Can you work these out from the drawing? Everything is in mm from the part's minimum corner. Round coordinates to 2 decimals unless told otherwise and drop trailing zeros. Order: outer loops, then holes, each group sorted by start corner. A loop starts at its lowest first (then second) coordinate and runs counter-clockwise, first axis right, second up. Notation, with made-up numbers: M 13.5,9.5 L 25.5,9.5 A15 cw 25.5,30.5 Z; hole C 62.25,70 d3. An arc over 180 degrees is marked long. Write item = value, one per line. Start each with the question number.
Item 1: I want a section at B-B, the plane x = 216. List the corners of the cut face in (y, z) for me.
Item 2: I want a section at C-C, the plane y = 1.8. List the corners of the cut face in (x, z) for me (3 decimals).
Item 3: I want a section at A-A, the plane z = 80. List the corners of the cut face in (x, y) for me (3 decimals), plus the area to 3 significant figures.
Item 4: I'm going to push flat-ended pins straight in: P1, Ø1.5, axis at x = 214.5, y = 2.5, coming from the +Z side; P2, Ø0.9, axis at x = 92.5, y = 2, coming from the +Z side. Where does each tip first touch, or does it pass through?
Item 5: I want a section at D-D, the plane x = 57.5. List the corners of the cut face in (y, z) for me, plus the area to 3 significant figures.
Item 6: Please list where these lines run through material, in increasing order: L1, parallel to X at y = 1.95, z = 80 (3 decimals); L2, parallel to Z at x = 141, y = 1; L3, parallel to Z at x = 189, y = 2.85.
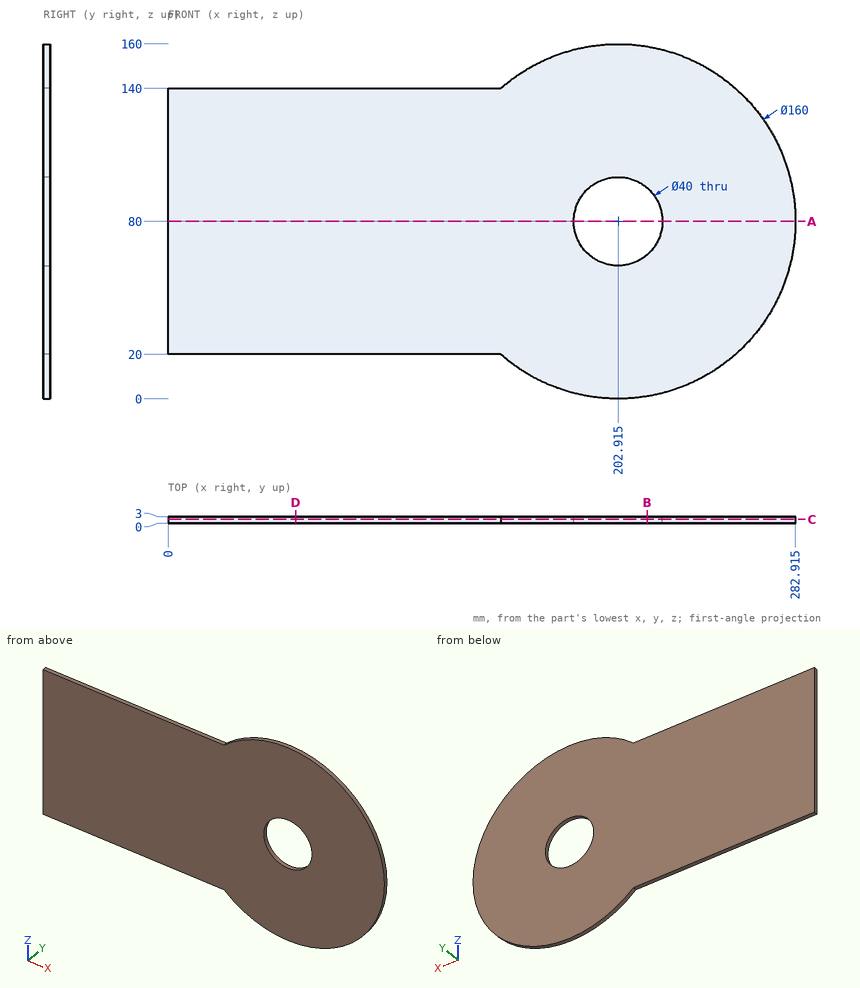
Filled in:
q1.outline = M 0,1.08 L 3,1.08 L 3,64.87 L 0,64.87 Z; M 0,95.13 L 3,95.13 L 3,158.92 L 0,158.92 Z
q2.outline = M 0,20 L 150,20 A80 ccw long 150,140 L 0,140 Z; hole C 202.915,80 d40
q3.outline = M 0,0 L 182.915,0 L 182.915,3 L 0,3 Z; M 222.915,0 L 282.915,0 L 282.915,3 L 222.915,3 Z
q3.area = 729 mm^2
q4.P1 = 159.26
q4.P2 = 140
q5.outline = M 0,20 L 3,20 L 3,140 L 0,140 Z
q5.area = 360 mm^2
q6.L1 = 0 to 182.915, 222.915 to 282.915
q6.L2 = 20 to 140
q6.L3 = 1.22 to 65.63, 94.37 to 158.78
